```python
from build123d import *

# Parameters (mm, degrees)
SKETCH1_W           = 21
SKETCH1_H           = 60
BOSS_EXTRUDE1_DEPTH = 12
BOSS_EXTRUDE2_DEPTH = 2.5
SKETCH7_R           = 1.6
CUT_EXTRUDE2_DEPTH  = 50.759421218


with BuildPart() as part:
    # Sketch1 → Boss-Extrude1 (new body)
    with BuildSketch(Plane(origin=(0, 0, 0), x_dir=(1, 0, 0), z_dir=(0, 1, 0))):
        Rectangle(SKETCH1_W, SKETCH1_H)
    extrude(amount=BOSS_EXTRUDE1_DEPTH)

    # Sketch2 → Cut-Revolve1 (revolve, cut)
    with BuildSketch(Plane(origin=(0, 12, 0), x_dir=(1, 0, 0), z_dir=(0, 1, 0))):
        Polygon((0, 30), (4.5, 30), (4.5, 27.5), (8, 27.5), (8, 23.25), (7.6, 23.25), (7.6, 22.25), (8, 22.25), (8, 7.75), (7.6, 7.75), (7.6, 6.75), (8, 6.75), (8, 2.5), (4.5, 2.5), (4.5, -2.5), (8, -2.5), (8, -6.75), (7.6, -6.75), (7.6, -7.75), (8, -7.75), (8, -22.25), (7.6, -22.25), (7.6, -23.25), (8, -23.25), (8, -27.5), (4.5, -27.5), (4.5, -30), (0, -30), align=None)
    revolve(axis=Axis((0, 12, 32.783592288), (0, 0, -1)), mode=Mode.SUBTRACT)

    # Sketch3 → Boss-Extrude2 (add)
    with BuildSketch(Plane.ZY.offset(10.5)):
        Polygon((-30, 0), (-30, 30), (-2.5, 30), (-2.5, 14), (18.5, 14), (18.5, 30), (30, 30), (30, 0), align=None)
    boss_extrude2 = extrude(amount=BOSS_EXTRUDE2_DEPTH)

    # Mirror2: Boss-Extrude2 across plane
    add(boss_extrude2.mirror(Plane(origin=(0, 0, 0), x_dir=(0, 0, 1), z_dir=(1, 0, 0))))

    # Sketch7 → Cut-Extrude2 (cut, through all)
    with BuildSketch(Plane.ZY.offset(13)):
        with Locations((22.5, 24)):
            Circle(SKETCH7_R)
        with Locations((-22.5, 24)):
            Circle(SKETCH7_R)
    extrude(amount=-CUT_EXTRUDE2_DEPTH, mode=Mode.SUBTRACT)


solid = part.part
```
Geometry check sheet. Reference: the model listing, model coordinates, mm. A direction names the side the tool comes from. Round coordinates to 2 decimals unless told otherwise and drop trailing zeros. Loops run counter-clockwise (first coordinate to the right, second up) from the corner with the lowest first, then second, coordinate; pieces in that order, holes last. Notation, with made-up numbers: M -28.75,70 L -20.75,70 A23 ccw -20.75,88 Z; hole C 71,88.25 d8. An arc over 180 degrees is marked long. Return JSON: item names as keys, results as strings. Group by question number.
(1) Mould release check, pull along Y, two halves, no side actions. Record for faces 4 (the face through (9, 12, 0)), 5 (the face through (11.733, 24.481, -20.974)), 6 (the face through (-12, 22, 18.5)): pulls with the +Y half, pulls with the -Y half, needs draft (parallel to the pull), parting line crosses it, or undercut.
(2) Section check C-C, the plane x = 0. Enter the section's corners in (y, z).
(3) Section check B-B, the plane y = 21. Enter the section's corners in (x, z), and give its area (3 significant figures).
(4) Section check A-A, the plane y = 24. Give the number of separate pieces and of enclosed holes in the cut face, and give its area (3 significant figures).
(5) Set-up check for faces 1 (the face through (-10.5, 21, -6)), 2 (the face through (0, 7, -2.5)), 3 (the face through (-12, 30, 24)): record each of +Z, -Z, +X, -X, +Y, -Y from which the full face is reachable in a straight line by a thin tool's end or side.
(6) Go/stop test with flat-tipped pins: pin 1 (1 mm diameter, centred on x = -1, z = -16, fed in from -Y); pin 2 (0.8 mm diameter, centred on x = -11, z = 4, fed in from +Y); pin 3 (5 mm diameter, centred on x = 7.5, z = 10, fed in from +Y). Record where each tip stops, or that it passes through.
(7) Section check D-D, the plane z = 15.5. Enter the section's corners in (x, y), and give its area (3 significant figures).
(8) Scan lines: line 1 along Z through (x, y) = (0, 7.25); line 2 along Y through (x, z) = (11.6, 22.5); line 3 along X through (y, z) = (23.5, -25). Record each from-to range of solid material in increasing order. Write a range as [from, to].
Data:
{
 "1": {"face 4": "pulls with the +Y half", "face 5": "undercut", "face 6": "needs draft"},
 "2": {"outline": "M 0,-30 L 7.5,-30 L 7.5,-27.5 L 4,-27.5 L 4,-23.25 L 4.4,-23.25 L 4.4,-22.25 L 4,-22.25 L 4,-7.75 L 4.4,-7.75 L 4.4,-6.75 L 4,-6.75 L 4,-2.5 L 7.5,-2.5 L 7.5,2.5 L 4,2.5 L 4,6.75 L 4.4,6.75 L 4.4,7.75 L 4,7.75 L 4,22.25 L 4.4,22.25 L 4.4,23.25 L 4,23.25 L 4,27.5 L 7.5,27.5 L 7.5,30 L 0,30 Z"},
 "3": {"outline": "M -13,-30 L -10.5,-30 L -10.5,-2.5 L -13,-2.5 Z; M -13,18.5 L -10.5,18.5 L -10.5,30 L -13,30 Z; M 10.5,-30 L 13,-30 L 13,-2.5 L 10.5,-2.5 Z; M 10.5,18.5 L 13,18.5 L 13,30 L 10.5,30 Z", "area": "195 mm²"},
 "4": {"separate pieces": "8", "enclosed holes": "0", "area": "163 mm²"},
 "5": {"face 1": "+Z, -Z, +Y", "face 2": "+Y", "face 3": "+Z, -Z, +X, -X, +Y"},
 "6": {"pin 1": "y = 0", "pin 2": "y = 14", "pin 3": "y = 12"},
 "7": {"outline": "M -13,0 L 13,0 L 13,14 L 10.5,14 L 10.5,12 L 8,12 A8 cw -8,12 L -10.5,12 L -10.5,14 L -13,14 Z", "area": "221 mm²"},
 "8": {"line 1": "[-30, -27.5], [-2.5, 2.5], [27.5, 30]", "line 2": "[0, 22.4], [25.6, 30]", "line 3": "[-13, -10.5], [10.5, 13]"}
}
